Here's how the part is built. I have some questions about the finished solid (model axes, mm). A direction names the side the tool comes from. Coordinates: 2 decimals unless noted, no trailing zeros. Write each loop counter-clockwise with the first axis right and the second up, starting at its lowest first coordinate (ties: lowest second). Pieces come first, ordered by that corner, then holes.
Item 1: I want a section at A-A (x = 2). Please give me the cut outline in (y, z).
Item 2: I want a section at C-C (z = -8.5). Please give me the cut outline in (x, y).
Item 3: If we mould it in two halves opening along X, with no side actions, what happens to faces 1 (the face through (17, -1256, 60.646)), 2 (the face through (44.544, -1256, -10)), 3 (the face through (16, -1256, -76.699))? For each: pulls with the +X half, pulls with the -X half, needs draft (parallel to the pull), parting line crosses it, or undercut.
Item 4: For faces 4 (the face through (43, -2438.4, -9)), 5 (the face through (16, -1256, 57.598)), which set-ups out of +Z, -Z, +X, -X, +Y, -Y let a thin tool reach every point of the face, with its end or its side?
Item 5: I want a section at B-B (y = -1557.5). Please give me the cut outline in (x, z) (1 decimal), and give its area (3 significant figures).
Item 6: I'm going to push flat-ended pins straight in: P1, Ø12, axis at y = -1443.5, z = 49, coming from the -X side; P2, Ø0.9, axis at x = -10.5, y = -1381.5, coming from the -Z side; P3, Ø10, axis at y = -1858.5, z = -49, coming from the -X side. Where does each tip first touch, or does it pass through?
Item 7: Please list where these lines run through material, in increasing order: line 1 (Z direction, x = 28.5, y = -1674); line 2 (X direction, y = -2045, z = -66.5); line 3 (X direction, y = -369.5, z = 51.5).
from build123d import *

# Parameters (mm, degrees)
F1_DEPTH = 2438.4
F2_W     = 49.059084
F2_H     = 106.4133
F3_DEPTH = 140.3941152
F4_R     = 3.175
F5_DEPTH = 3.302


with BuildPart() as f1:
    # F0 (on Front) → F1 (new body)
    with BuildSketch(Plane.XZ):
        with BuildLine():
            Line((-10.5452926, -75.1112544), (-10.5452926, -60.6967544))
            Line((-10.5452926, -60.6967544), (-13.5932926, -60.6967544))
            Line((-13.5932926, -60.6967544), (-13.5932926, -75.1112544))
            ThreePointArc((-13.5932926, -75.1112544), (-12.2355860842, -78.3890478842), (-8.9577926, -79.7467544))
            Line((-8.9577926, -79.7467544), (40.7343864, -79.7467544))
            ThreePointArc((40.7343864, -79.7467544), (43.4284632363, -78.6308312363), (44.5443864, -75.9367544))
            Line((44.5443864, -75.9367544), (44.5443864, 56.8363608))
            ThreePointArc((44.5443864, 56.8363608), (43.4284632363, 59.5304376363), (40.7343864, 60.6463608))
            Line((40.7343864, 60.6463608), (-8.3246976, 60.6463608))
            ThreePointArc((-8.3246976, 60.6463608), (-11.0187744363, 59.5304376363), (-12.1346976, 56.8363608))
            Line((-12.1346976, 56.8363608), (-12.1346976, 41.5963608))
            Line((-12.1346976, 41.5963608), (-9.0866976, 41.5963608))
            Line((-9.0866976, 41.5963608), (-9.0866976, 56.8363608))
            ThreePointArc((-9.0866976, 56.8363608), (-8.8635129673, 57.3751761673), (-8.3246976, 57.5983608))
            Line((-8.3246976, 57.5983608), (40.7343864, 57.5983608))
            ThreePointArc((40.7343864, 57.5983608), (41.2732017673, 57.3751761673), (41.4963864, 56.8363608))
            Line((41.4963864, 56.8363608), (41.4963864, -75.9367544))
            ThreePointArc((41.4963864, -75.9367544), (41.2732017673, -76.4755697673), (40.7343864, -76.6987544))
            Line((40.7343864, -76.6987544), (-8.9577926, -76.6987544))
            ThreePointArc((-8.9577926, -76.6987544), (-10.0803246151, -76.2337864151), (-10.5452926, -75.1112544))
        make_face()
    extrude(amount=F1_DEPTH)

    # F2 (on face) → F3 (cut, through all)
    with BuildSketch(Plane.XY.offset(60.6463608)):
        Polygon((-56.2798976, -106.4133), (-8.3246976, -106.4133), (-8.3246976, 0), (40.7343864, 0), (40.7343864, -106.4133), (92.9059864, -106.4133), (92.9059864, 23.1394), (-56.2798976, 23.1394), align=None)
        with Locations((16.2048444, -53.20665)):
            Rectangle(F2_W, F2_H)
    extrude(amount=-F3_DEPTH, mode=Mode.SUBTRACT)

    # F4 (on face) → F5 (cut)
    with BuildSketch(Plane.XY.offset(60.6463608)):
        with Locations((16.2048444, -134.3406)):
            Circle(F4_R)
        with Locations((16.2048444, -589.407)):
            Circle(F4_R)
        with Locations((16.2048444, -1044.4734)):
            Circle(F4_R)
        with Locations((16.2048444, -1499.5398)):
            Circle(F4_R)
        with Locations((16.2048444, -1954.6062)):
            Circle(F4_R)
    extrude(amount=-F5_DEPTH, mode=Mode.SUBTRACT)


solid = f1.part
Answer:
1. outline: (-2438.4, -79.75) - (-106.41, -79.75) - (-106.41, -76.7) - (-2438.4, -76.7) - close; (-2438.4, 57.6) - (-106.41, 57.6) - (-106.41, 60.65) - (-2438.4, 60.65) - close
2. outline: (41.5, -2438.4) - (44.54, -2438.4) - (44.54, -106.41) - (41.5, -106.41) - close
3. face 1: needs draft
3. face 2: pulls with the +X half
3. face 3: undercut
4. face 4: +Z, -Z, +X, -X, -Y
4. face 5: +Y, -Y
5. outline: (-13.6, -75.1) arc R4.6 ccw to (-9, -79.7) - (40.7, -79.7) arc R3.8 ccw to (44.5, -75.9) - (44.5, 56.8) arc R3.8 ccw to (40.7, 60.6) - (-8.3, 60.6) arc R3.8 ccw to (-12.1, 56.8) - (-12.1, 41.6) - (-9.1, 41.6) - (-9.1, 56.8) arc R0.8 cw to (-8.3, 57.6) - (40.7, 57.6) arc R0.8 cw to (41.5, 56.8) - (41.5, -75.9) arc R0.8 cw to (40.7, -76.7) - (-9, -76.7) arc R1.6 cw to (-10.5, -75.1) - (-10.5, -60.7) - (-13.6, -60.7) - close
5. area: 844 mm2
6. P1: stops at x = -12.13
6. P2: stops at z = -79.62
6. P3: stops at x = 41.5
7. line 1: z = -79.75 to -76.7, 57.6 to 60.65
7. line 2: x = -13.59 to -10.55, 41.5 to 44.54
7. line 3: x = -12.13 to -9.09, 41.5 to 44.54
